CAD build for the part. Positions are in the model's coordinates, mm. A direction names the side the tool comes from. Coordinates: 2 decimals unless noted, no trailing zeros. Loops run counter-clockwise (first coordinate to the right, second up) from the corner with the lowest first, then second, coordinate; pieces in that order, holes last. Notation, with made-up numbers: (-22.75, -17) -> (1.25, -17) arc R36 cw to (1.25, 20) -> close; hole circle Ø6 at (0.5, -32). An arc over 180 degrees is marked (long way). Write item = value, one per line. Start each with the question number.
(1) Band-saw the part on B-B (y = 36). Write the cut outline in (x, z).
(2) Band-saw the part on C-C (x = 20.5). Write the cut outline in (y, z), and give its area (3 significant figures).
(3) Pull direction X, two halves, no side cores. Call faces 1 (the face through (32.68, 25.64, 58.94)), 2 (the face through (25.483, 36.121, 58.939)), 3 (the face through (6.645, 28.379, 58.939)): +X half, -X half, draft (parallel to the pull), parting line (faces both ways), or undercut.
(4) Drill centre lines: line 1 (Y direction, x = 30.5, z = 64); line 2 (Y direction, x = 29.5, z = 52.75); line 3 (X direction, y = 33.5, z = 54). Where is each one in solid material? Low to high. Write a range as from..to.
(5) Flat gauge pins, fed straight in: P1, Ø1, axis at y = 30, z = 62.5, coming from the +X side; P2, Ø8, axis at y = 29, z = 60, coming from the +X side; P3, Ø3, axis at y = 17.5, z = 60, coming from the +X side. Where does each tip first touch, or does it go through?
(6) Band-saw the part on D-D (y = 25). Write the cut outline in (x, z), and give its area (3 significant figures).
(7) Band-saw the part on A-A (z = 55.75). Write the cut outline in (x, y).
(8) Tool access for faces 4 (the face through (14.8, 13.2, 58.9)), 5 (the face through (28.75, 34.16, 58.94)), 6 (the face through (29.502, 10.553, 58.939)), 7 (the face through (13.623, 38.396, 58.939)), 8 (the face through (19, 24, 50.8)): list every direction of +Z, -Z, +X, -X, +Y, -Y with a clear straight run to the whole face (end or side of a thin tool).
```python
from build123d import *

# Parameters (mm, degrees)
SKETCH1_W      = 203.2
SKETCH1_H      = 101.6
EXTRUDE1_DEPTH = 50.8
EXTRUDE2_DEPTH = 16.51
SKETCH23_W     = 203.2
SKETCH23_H     = 50.8
EXTRUDE3_DEPTH = 508


with BuildPart() as part:
    # Sketch1 → Extrude1 (new body)
    with BuildSketch(Plane.XY):
        with Locations((101.6, 50.8)):
            Rectangle(SKETCH1_W, SKETCH1_H)
    extrude(amount=EXTRUDE1_DEPTH)

    # Sketch21 → Extrude2 (add)
    with BuildSketch(Plane.XY.offset(50.8)):
        Polygon((10.680914086, 39.466921448), (16.647962228, 37.295093538), (23.464694461, 32.952356157), (27.558917476, 39.378998974), (30.772238885, 37.331887466), (26.678015869, 30.905244649), (33.104658686, 26.811021633), (32.238976379, 24.432579042), (36.293520259, 22.947359397), (31.515498857, 9.819853485), (27.43078785, 11.306566707), (26.589174956, 8.909877207), (2.720982388, 17.597188848), align=None)
    extrude(amount=EXTRUDE2_DEPTH)

    # Sketch23 → Extrude3 (cut)
    with BuildSketch(Plane.XZ):
        with Locations((101.6, 25.4)):
            Rectangle(SKETCH23_W, SKETCH23_H)
    extrude(amount=-EXTRUDE3_DEPTH, mode=Mode.SUBTRACT)


solid = part.part
```
Findings below:
q1.outline = (9.42, 50.8) -> (18.68, 50.8) -> (18.68, 67.31) -> (9.42, 67.31) -> close; (25.41, 50.8) -> (29.92, 50.8) -> (29.92, 67.31) -> (25.41, 67.31) -> close
q2.outline = (11.13, 50.8) -> (34.84, 50.8) -> (34.84, 67.31) -> (11.13, 67.31) -> close
q2.area = 392 mm²
q3.face_1 = +X half
q3.face_2 = undercut
q3.face_3 = -X half
q4.line_1 = 10.19..28.47, 36.9..37.51
q4.line_2 = 10.55..29.11, 35.33..38.14
q4.line_3 = 8.51..22.61, 23.81..28.33
q5.P1 = 28.88
q5.P2 = 33.1
q5.P3 = 34.86
q6.outline = (5.42, 50.8) -> (32.45, 50.8) -> (32.45, 67.31) -> (5.42, 67.31) -> close
q6.area = 446 mm²
q7.outline = (2.72, 17.6) -> (26.59, 8.91) -> (27.43, 11.31) -> (31.52, 9.82) -> (36.29, 22.95) -> (32.24, 24.43) -> (33.1, 26.81) -> (26.68, 30.91) -> (30.77, 37.33) -> (27.56, 39.38) -> (23.46, 32.95) -> (16.65, 37.3) -> (10.68, 39.47) -> close
q8.face_4 = +Z, -Z, -X, -Y
q8.face_5 = +Z, -Z, +X
q8.face_6 = +Z, -Z, -Y
q8.face_7 = +Z, -Z, +Y
q8.face_8 = -Z, +X, -X, +Y, -Y
